Part model, mm, in its own coordinate system. A direction names the side the tool comes from. Coordinates: 2 decimals unless noted, no trailing zeros. Order: outer loops, then holes, each group sorted by start corner. A loop starts at its lowest first (then second) coordinate and runs counter-clockwise, first axis right, second up. Notation, with made-up numbers: (-2.5, 9) - (40.5, 9) arc R20 cw to (40.5, 36) - close; hole circle Ø11 at (59, 61.25). An arc over 180 degrees is marked (long way). Use a Markdown table: item, result. Add a question column.
1) Wall check: L1, parallel to X at y = 37, z = 2; L2, parallel to Y at x = -74.75, z = 6.25; L3, parallel to Y at x = -75.75, z = 4.25. Give the ranges that are in metal, low to high. Write a range as [from, to].
2) Saw through at C-C on x = -64. List the corners of the cut face in (y, z), then the cut area to 3 significant figures.
3) Saw through at B-B on y = 36.5. List the corners of the cut face in (x, z), then the cut area to 3 significant figures.
4) Tool access for faces 4 (the face through (-76.857, 10.355, 2.465)), 5 (the face through (-66.566, 37.635, 3.944)): list every direction of +Z, -Z, +X, -X, +Y, -Y with a clear straight run to the whole face (end or side of a thin tool).
5) Saw through at A-A on z = 3. List the corners of the cut face in (x, y), then the cut area to 3 significant figures.
6) Saw through at D-D on z = 8.5. List the corners of the cut face in (x, y), then the cut area to 3 significant figures.
7) Two-plate mould, pull along Y, no slides. Class faces 1 (the face through (-63.468, 44.353, 10.846)), 2 (the face through (-71.12, 26.558, 13.381)), 3 (the face through (-76.22, 20.63, 3.94)): +Y half, -Y half, draft (parallel to the pull), parting line (faces both ways), or undercut.
8) Drop flat-ended pins along their axis: P1, Ø3, axis at x = -76, z = 14, coming from the +Y side; P2, Ø2.5, axis at x = -74.72, y = 20.56, coming from the +Z side; P3, Ø12, axis at y = 17.5, z = 13.5, coming from the +X side. Give the stop position or say it passes through.
```python
from build123d import *

# Parameters (mm, degrees)
F0_R        = 1.5
F1_DEPTH    = 22
F2_T1_DEPTH = 165.8159550338
F3_DEPTH    = 8


# Not quite as in the source:
# - a fillet or chamfer that OpenCascade refuses, or shapes differently, is made with other operations: its cross-section is extruded or revolved along the edge and cut away or added


with BuildPart() as f1:
    # F0 (on Top) → F1 (new body)
    with BuildSketch(Plane.XY):
        with BuildLine():
            ThreePointArc((-71.5091042417, 11.9456272565), (-71.2779515077, 13.2553245479), (-71.0228136012, 14.5605613962))
            Line((-71.0228136012, 14.5605613962), (-78.4331581972, 13.1022935094))
            Line((-78.4331581972, 13.1022935094), (-71.5091042417, 11.9456272565))
        make_face()
        with BuildLine():
            ThreePointArc((-71.0228136012, 14.5605613962), (-66.9578457789, 27.8010231583), (-60.4491628751, 40.0268498348))
            Line((-60.4491628751, 40.0268498348), (-68.7869784441, 45.5477946397))
            ThreePointArc((-68.7869784441, 45.5477946397), (-76.7608906967, 30.2326918988), (-81.3724289647, 13.5932999815))
            Line((-81.3724289647, 13.5932999815), (-78.4331581972, 13.1022935094))
            Line((-78.4331581972, 13.1022935094), (-71.0228136012, 14.5605613962))
        make_face()
        with Locations((-74.7222680365, 20.5628952117)):
            Circle(F0_R, mode=Mode.SUBTRACT)
        with Locations((-67.9969340878, 37.184229919)):
            Circle(F0_R, mode=Mode.SUBTRACT)
        with BuildLine():
            ThreePointArc((-60.4491628751, 40.0268498348), (-59.9428373222, 40.7811997588), (-59.4270987125, 41.5291456523))
            Line((-59.4270987125, 41.5291456523), (-67.6239399142, 47.2573036734))
            ThreePointArc((-67.6239399142, 47.2573036734), (-68.2108148839, 46.4061928289), (-68.7869784441, 45.5477946397))
            Line((-68.7869784441, 45.5477946397), (-60.4491628751, 40.0268498348))
        make_face()
        with BuildLine():
            ThreePointArc((-71.5997882434, 11.3894830218), (-71.554986557, 11.667643242), (-71.5091042417, 11.9456272565))
            Line((-71.5091042417, 11.9456272565), (-78.4331581972, 13.1022935094))
            Line((-78.4331581972, 13.1022935094), (-81.5492033125, 12.4890928052))
            ThreePointArc((-81.5492033125, 12.4890928052), (-81.7739574871, 10.9210748966), (-81.9685648448, 9.3490308206))
            Line((-81.9685648448, 9.3490308206), (-71.5997882434, 11.3894830219))
        make_face()
        with BuildLine():
            Line((-81.5492033125, 12.4890928052), (-78.4331581972, 13.1022935094))
            Line((-78.4331581972, 13.1022935094), (-81.3724289647, 13.5932999815))
            ThreePointArc((-81.3724289647, 13.5932999815), (-81.462687068, 13.0414959135), (-81.5492033125, 12.4890928052))
        make_face()
        with Locations((-67.9969340878, 37.184229919)):
            Circle(F0_R)
        with Locations((-74.7222680365, 20.5628952117)):
            Circle(F0_R)
    extrude(amount=F1_DEPTH)

    # F2: chamfer of 17 x 30 on 1 edges, made by hand

    # F2_s2 → F2_t1 (cut)
    with BuildSketch(Plane(origin=(-153.3048702431, -30.1685793773, 0), x_dir=(0, 0, 1), z_dir=(0.9811820369, 0.1930849823, 0))):
        Polygon((5, -25), (22, -55), (22, -25), align=None)
    extrude(amount=F2_T1_DEPTH, mode=Mode.SUBTRACT)

    # F0 (on Top) → F3 (cut)
    with BuildSketch(Plane.XY):
        with Locations((-67.9969340878, 37.184229919)):
            Circle(F0_R)
        with Locations((-74.7222680365, 20.5628952117)):
            Circle(F0_R)
    extrude(amount=F3_DEPTH, mode=Mode.SUBTRACT)


solid = f1.part
```
Results are:
| question | item | result |
|---|---|---|
| 1 | L1 | [-73.74, -69.49], [-66.51, -62.35] |
| 1 | L2 | [13.02, 19.06], [22.06, 34.91] |
| 1 | L3 | [10.57, 19.47], [21.66, 32.68] |
| 2 | outline | (34.06, 0) - (44.72, 0) - (44.72, 22) - (43.46, 22) - (34.06, 16.77) - close |
| 2 | area | 210 mm2 |
| 3 | outline | (-73.99, 0) - (-69.33, 0) - (-69.33, 8) - (-66.66, 8) - (-66.66, 0) - (-62.64, 0) - (-62.64, 17.98) - (-73.99, 19.22) - close |
| 3 | area | 190 mm2 |
| 4 | face 4 | +Z, -Z, +X, -Y |
| 4 | face 5 | -Z |
| 5 | outline | (-81.97, 9.35) - (-71.6, 11.39) arc R72.5 cw to (-71.51, 11.95) arc R72.5 cw to (-59.43, 41.53) - (-67.62, 47.26) arc R82.5 ccw to start; hole circle Ø3 at (-74.72, 20.56); hole circle Ø3 at (-68, 37.18) |
| 5 | area | 355 mm2 |
| 6 | outline | (-80.96, 15.84) - (-70.24, 17.95) arc R72.5 cw to (-59.43, 41.53) - (-67.62, 47.26) arc R82.5 ccw to start |
| 6 | area | 302 mm2 |
| 7 | face 1 | +Y half |
| 7 | face 2 | -Y half |
| 7 | face 3 | undercut |
| 8 | P1 | y = 35.44 |
| 8 | P2 | z = 11.15 |
| 8 | P3 | x = -68.75 |
